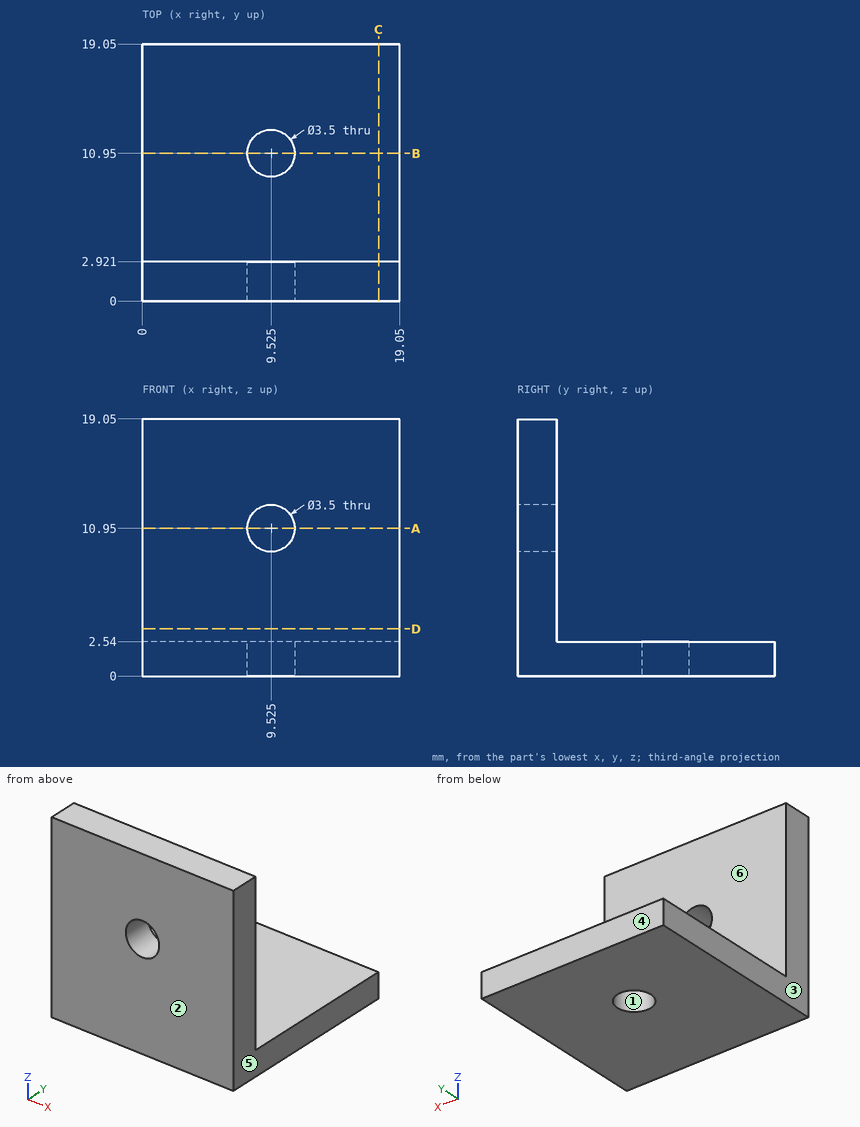
The figure shows three views and two pictorial views of one solid part (mm, origin at its lowest corner). Answer the questions. A direction names the side the tool comes from. Round coordinates to 2 decimals unless told otherwise and drop trailing zeros. Write each loop counter-clockwise with the first axis right and the second up, starting at its lowest first coordinate (ties: lowest second). Pieces come first, ordered by that corner, then holes. Notation, with made-up numbers: (63.25, 5) -> (112.25, 5) arc R15 ccw to (112.25, 16) -> close; hole circle Ø2 at (74.25, 40.25). An arc over 180 degrees is marked (long way). Answer as a JSON object with one key per item and string values. Group by question number.
Q1. Determine the mould class of the marked faces 1, 2, 3 and 4 for opening direction Y: pulls with the +Y half, pulls with the -Y half, needs draft (parallel to the pull), parting line crosses it, or undercut.
Q2. Straight lines are drawn through the part: line 1 along Y through (x, z) = (18, 15.75); line 2 along Z through (x, y) = (1.5, 11); line 3 along X through (y, z) = (1, 11.25). For each, find the intervals that lie inside material, in ascending order.
Q3. Section C-C (x = 17.5) is taken. Write down the section's boundary in (y, z), plus the area to 3 significant figures.
Q4. Each of these flat-tipped pins is pushed along its axis until it touches: pin 1 Ø5 at (x, y) = (9.5, 7) entering from -Z; pin 2 Ø4 at (x, z) = (11.5, 13) entering from +Y. Where does it stop, or does it pass through?
Q5. Which of the six approach directions +Z, -Z, +X, -X, +Y, -Y give full straight-line access (tool end or side, diameter ignored) to the marked faces 5 and 6?
Q6. Section A-A (z = 10.95) is taken. Write down the section's boundary in (x, y) (3 decimals), plus the area to 3 significant figures.
Q7. Section B-B (y = 10.95) is taken. Write down the section's boundary in (x, z) (3 decimals), plus the area to 3 significant figures.
Q8. Section D-D (z = 3.5) is taken. Write down the section's boundary in (x, y).
Check values:
{
 "1": {"face 1": "undercut", "face 2": "pulls with the -Y half", "face 3": "needs draft", "face 4": "pulls with the +Y half"},
 "2": {"line 1": "0 to 2.92", "line 2": "0 to 2.54", "line 3": "0 to 7.8, 11.25 to 19.05"},
 "3": {"outline": "(0, 0) -> (19.05, 0) -> (19.05, 2.54) -> (2.92, 2.54) -> (2.92, 19.05) -> (0, 19.05) -> close", "area": "96.6 mm^2"},
 "4": {"pin 1": "z = 0", "pin 2": "y = 2.92"},
 "5": {"face 5": "+Z, -Z, +X, +Y, -Y", "face 6": "+Z, +X, -X, +Y"},
 "6": {"outline": "(0, 0) -> (7.775, 0) -> (7.775, 2.921) -> (0, 2.921) -> close; (11.275, 0) -> (19.05, 0) -> (19.05, 2.921) -> (11.275, 2.921) -> close", "area": "45.4 mm^2"},
 "7": {"outline": "(0, 0) -> (7.775, 0) -> (7.775, 2.54) -> (0, 2.54) -> close; (11.275, 0) -> (19.05, 0) -> (19.05, 2.54) -> (11.275, 2.54) -> close", "area": "39.5 mm^2"},
 "8": {"outline": "(0, 0) -> (19.05, 0) -> (19.05, 2.92) -> (0, 2.92) -> close"}
}
